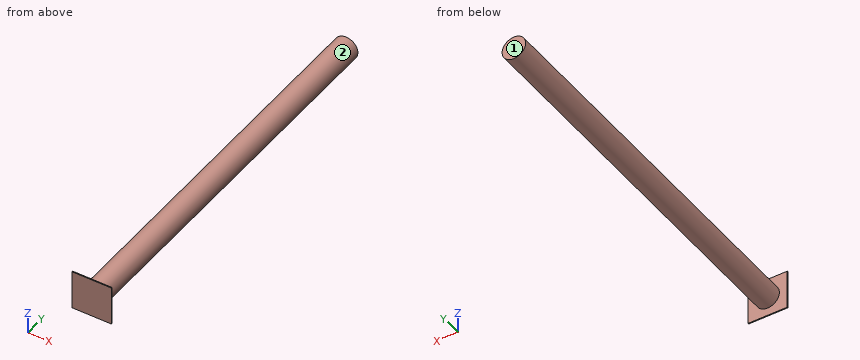
```python
from build123d import *

# Parameters (mm, degrees)
SKETCH_1_R      = 60
EXTRUDE_1_DEPTH = 2000
SKETCH_2_W      = 200
SKETCH_2_H      = 200
EXTRUDE_2_DEPTH = 5


with BuildPart() as part:
    # 草圖1 → 填料-伸長1 (new body)
    with BuildSketch(Plane(origin=(0, 0, 0), x_dir=(1, 0, 0), z_dir=(0, 1, 0))):
        Circle(SKETCH_1_R)
    extrude(amount=EXTRUDE_1_DEPTH)

    # 草圖2 → 填料-伸長2 (add)
    with BuildSketch(Plane.XZ):
        Rectangle(SKETCH_2_W, SKETCH_2_H)
    extrude(amount=-EXTRUDE_2_DEPTH)


solid = part.part
```
Build history of the part. All positions in model axes, mm. Face numbers are marked on the shaded views. A direction names the side the tool comes from. Give positions to 0.01 mm unless a question says otherwise; leave off trailing zeros. Loops run counter-clockwise (first coordinate to the right, second up) from the corner with the lowest first, then second, coordinate; pieces in that order, holes last.
Item 1: Slice it at B-B, the plane z = -36. List the corners of the cut face in (x, y).
Answers follow:
outline: (-100, 0) - (100, 0) - (100, 5) - (48, 5) - (48, 2000) - (-48, 2000) - (-48, 5) - (-100, 5) - close
Item 2: Slice it at A-A, the plane x = 0. List the corners of the cut face in (y, z), and give its area (3 significant figures).
Answers follow:
outline: (0, -100) - (5, -100) - (5, -60) - (2000, -60) - (2000, 60) - (5, 60) - (5, 100) - (0, 100) - close
area: 240,000 mm2
Item 3: Which spindle directions (+Z, -Z, +X, -X, +Y, -Y) get a long thin tool onto all of the face, cutting with end or side? Do the marked faces 1 and 2. Say none if no direction does.
Answers follow:
face 1: +Z, -Z, +X, -X, +Y
face 2: +Y
Item 4: Slice it at C-C, the plane y = 648.5. List the corners of the cut face in (x, z).
Answers follow:
outline: circle Ø120 at (0, 0)
Item 5: Flat gauge pins, fed straight in: pin 1 (6 mm diameter, centred on x = 54, y = 577, fed in from +Z); pin 2 (6 mm diameter, centred on x = -52, y = 1635, fed in from +Z); pin 3 (1 mm diameter, centred on y = 700, z = 35.5, fed in from -X). Where does each tip first touch, or does it go through?
Answers follow:
pin 1: stops at z = 31.61
pin 2: stops at z = 34.63
pin 3: stops at x = -48.73
Item 6: Drill centre lines: line 1 (Y direction, x = 65, z = 87.5); line 2 (X direction, y = 926.5, z = 0.5); line 3 (X direction, y = 1861, z = -8). Where is each one in solid material? Low to high.
Answers follow:
line 1: y = 0 to 5
line 2: x = -60 to 60
line 3: x = -59.46 to 59.46
